The model under review builds one solid part; all positions refer to its coordinate system, in mm. Face numbers are marked on the shaded views. Round coordinates to 2 decimals unless told otherwise and drop trailing zeros. Order: outer loops, then holes, each group sorted by start corner. A loop starts at its lowest first (then second) coordinate and runs counter-clockwise, first axis right, second up. Notation, with made-up numbers: (-36.5, -36.75) -> (13.5, -36.75) arc R32 cw to (13.5, -2.75) -> close; hole circle Ø10 at (24.25, 47.5). An arc over 180 degrees is marked (long way). Return JSON: item names as keys, results as strings. Group by question number.
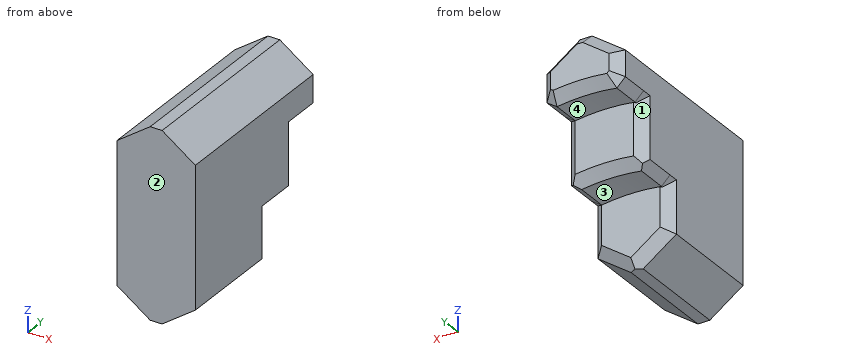
from build123d import *

# Parameters (mm, degrees)
EXTRUDE1_DEPTH     = 9.9822
CUT_EXTRUDE1_DEPTH = 36.749577377
SKETCH3_R          = 25.885731189
CUT_EXTRUDE2_DEPTH = 4.9022
SKETCH4_R          = 25.885731189
CUT_EXTRUDE3_DEPTH = 5.2578
CHAMFER1_SIZE      = 1.08172717
CHAMFER1_SIZE_2    = 1.27
CHAMFER2_SIZE      = 1.27
CHAMFER3_SIZE      = 1.27
CHAMFER4_SIZE      = 1.27


with BuildPart() as part:
    # Sketch1 → Extrude1 (new body)
    with BuildSketch(Plane(origin=(0, 0, 0), x_dir=(0, 0, -1), z_dir=(1, 0, 0))):
        Polygon((7.5692, 24.6888), (7.5692, 19.7866), (15.4432, 19.7866), (15.4432, 14.5288), (23.8506, 14.5288), (23.8506, 0), (0, 0), (0, 24.6888), align=None)
    extrude(amount=EXTRUDE1_DEPTH)

    # Sketch2 → Cut-Extrude1 (cut, through all)
    with BuildSketch(Plane(origin=(0, 24.6888, 0), x_dir=(1, 0, 0), z_dir=(0, 1, 0))):
        Polygon((0, 2.9972), (4.2291, 0), (0, 0), align=None)
        Polygon((9.9822, 2.9972), (9.9822, 0), (5.7531, 0), align=None)
        Polygon((0, 23.8506), (4.2291, 23.8506), (0, 20.8534), align=None)
        Polygon((9.9822, 20.8534), (9.9822, 23.8506), (5.7531, 23.8506), align=None)
    extrude(amount=-CUT_EXTRUDE1_DEPTH, mode=Mode.SUBTRACT)

    # Sketch3 → Cut-Extrude2 (cut)
    with BuildSketch(Plane(origin=(0, 24.6888, 0), x_dir=(1, 0, 0), z_dir=(0, 1, 0))):
        with Locations((4.9911, 32.9692)):
            Circle(SKETCH3_R)
    extrude(amount=-CUT_EXTRUDE2_DEPTH, mode=Mode.SUBTRACT)

    # Sketch4 → Cut-Extrude3 (cut)
    with BuildSketch(Plane(origin=(0, 19.7866, 0), x_dir=(1, 0, 0), z_dir=(0, 1, 0))):
        with Locations((4.9911, 40.8432)):
            Circle(SKETCH4_R)
    extrude(amount=-CUT_EXTRUDE3_DEPTH, mode=Mode.SUBTRACT)

    # Chamfer1
    # the kernel refuses this chamfer: 1.27, 1.08172717 mm, written as the material it takes off along each edge
    with BuildSketch(Plane(origin=(9.9822, 23.137823144, -15.4432), x_dir=(-0.9857782143008734, 0, 0.168051516535202), z_dir=(0, -1, 0))) as chamfer1_piece_1:
        with BuildLine():
            Line((1.303218251, 0), (CHAMFER1_SIZE * 0.168051516609, -CHAMFER1_SIZE * 0.985778214731))
            Line((CHAMFER1_SIZE * 0.168051516609, -CHAMFER1_SIZE * 0.985778214731), (0, 0))
            ThreePointArc((0, 0), (0.67003435, -0.008196065), (1.303218251, 0))
        make_face()
    extrude(amount=8.609023144, mode=Mode.SUBTRACT)
    with BuildSketch(Plane(origin=(9.9822, 28.040023144, -7.5692), x_dir=(0, 0, 1), z_dir=(0, -1, 0))) as chamfer1_piece_2:
        with BuildLine():
            Line((CHAMFER1_SIZE, 0), (0.219007803, 1.28468416))
            ThreePointArc((0.219007803, 1.28468416), (0.12067979, 0.659127904), (0, 0))
            Line((0, 0), (CHAMFER1_SIZE, 0))
        make_face()
    extrude(amount=8.253423144, mode=Mode.SUBTRACT)
    with BuildSketch(Plane(origin=(0, 27.954837395, -7.5692), x_dir=(0.9851028173062452, 0, 0.1719663901327771), z_dir=(0, -1, 0))) as chamfer1_piece_3:
        with BuildLine():
            Line((1.097600724, 0), (CHAMFER1_SIZE_2 * 0.171966390133, CHAMFER1_SIZE_2 * 0.985102817306))
            Line((CHAMFER1_SIZE_2 * 0.171966390133, CHAMFER1_SIZE_2 * 0.985102817306), (0, 0))
            ThreePointArc((0, 0), (0.563419729, 0.005814052), (1.097600724, 0))
        make_face()
    extrude(amount=8.168237395, mode=Mode.SUBTRACT)
    with BuildSketch(Plane(origin=(0, 23.052637395, -15.4432), x_dir=(0.985102817306246, 0, 0.17196639013277196), z_dir=(0, -1, 0))) as chamfer1_piece_4:
        with BuildLine():
            Line((1.097600724, 0), (CHAMFER1_SIZE_2 * 0.171966390133, CHAMFER1_SIZE_2 * 0.985102817306))
            Line((CHAMFER1_SIZE_2 * 0.171966390133, CHAMFER1_SIZE_2 * 0.985102817306), (0, 0))
            ThreePointArc((0, 0), (0.563419729, 0.005814052), (1.097600724, 0))
        make_face()
    extrude(amount=8.523837395, mode=Mode.SUBTRACT)

    # Chamfer2
    # the kernel refuses this chamfer: 1.27 mm, written as the material it takes off along each edge
    with BuildSketch(Plane(origin=(3.088405412, 24.6888, 1.88849226), x_dir=(0, -1, 0), z_dir=(0.8158799994392605, 0, -0.5782212608638604))) as chamfer2_piece_1:
        Polygon((CHAMFER2_SIZE, 0), (0, CHAMFER2_SIZE), (0, 0), align=None)
    extrude(amount=11.715557658, mode=Mode.SUBTRACT)
    with BuildSketch(Plane(origin=(0.963062605, 24.6888, 0), x_dir=(0, 0, -1), z_dir=(1, 0, 0))) as chamfer2_piece_2:
        Polygon((CHAMFER2_SIZE, 0), (0, -CHAMFER2_SIZE), (0, 0), align=None)
    extrude(amount=8.056074789, mode=Mode.SUBTRACT)
    with BuildSketch(Plane(origin=(-2.664694588, 24.6888, -4.88569226), x_dir=(0.5782212608638604, 0, -0.8158799994392603), z_dir=(0.8158799994392604, 0, 0.5782212608638605))) as chamfer2_piece_3:
        Polygon((CHAMFER2_SIZE, 0), (0, -CHAMFER2_SIZE), (0, 0), align=None)
    extrude(amount=11.715557658, mode=Mode.SUBTRACT)
    with BuildSketch(Plane(origin=(0, 24.6888, 0.268837395), x_dir=(1, 0, 0), z_dir=(0, 0, -1))) as chamfer2_piece_4:
        Polygon((CHAMFER2_SIZE, 0), (0, CHAMFER2_SIZE), (0, 0), align=None)
    extrude(amount=9.834074789, mode=Mode.SUBTRACT)
    with BuildSketch(Plane(origin=(3.390686755, 24.6888, -9.689886755), x_dir=(0.7071067811864264, 0, 0.7071067811866687), z_dir=(-0.7071067811866687, 0, 0.7071067811864264))) as chamfer2_piece_5:
        Polygon((CHAMFER2_SIZE, 0), (0, -CHAMFER2_SIZE), (0, 0), align=None)
    extrude(amount=8.061192589, mode=Mode.SUBTRACT)
    with BuildSketch(Plane(origin=(4.9911, 24.6888, -32.9692), x_dir=(-0.27423691753181434, 0, 0.9616621616049208), z_dir=(-0.9616621616049208, 0, -0.27423691753181434))) as chamfer2_piece_6:
        Polygon((25.885731189 + CHAMFER2_SIZE, 0), (25.885731189, -CHAMFER2_SIZE), (25.885731189, 0), align=None)
    revolve(axis=Axis((4.9911, 24.6888, -32.9692), (0, 1, 0)), revolution_arc=31.377850279, mode=Mode.SUBTRACT)
    with BuildSketch(Plane(origin=(12.693590923, 24.6888, -4.666659955), x_dir=(-0.5574990899678705, 0, 0.8301775500969635), z_dir=(-0.8301775500969636, 0, -0.5574990899678705))) as chamfer2_piece_7:
        Polygon((CHAMFER2_SIZE, 0), (0, -CHAMFER2_SIZE), (0, 0), align=None)
    extrude(amount=8.079556, mode=Mode.SUBTRACT)
    with BuildSketch(Plane(origin=(9.9822, 24.6888, 0.268837395), x_dir=(-1, 0, 0), z_dir=(0, 0, -1))) as chamfer2_piece_8:
        Polygon((CHAMFER2_SIZE, 0), (0, -CHAMFER2_SIZE), (0, 0), align=None)
    extrude(amount=10.022347619, mode=Mode.SUBTRACT)
    with BuildSketch(Plane(origin=(9.9822, 14.5288, -24.119437395), x_dir=(-1, 0, 0), z_dir=(0, 0, 1))) as chamfer2_piece_9_section:
        Polygon((CHAMFER2_SIZE, 0), (0, CHAMFER2_SIZE), (0, 0), align=None)
    chamfer2_piece_9 = extrude(amount=13.02400196, mode=Mode.PRIVATE)
    chamfer2_piece_9 = split(chamfer2_piece_9, bisect_by=Plane(origin=(5.465987334, 14.5288, -17.394299305), z_dir=(0.5574990901783627, 0, -0.8301775499556092)), keep=Keep.TOP, mode=Mode.PRIVATE)
    add(chamfer2_piece_9, mode=Mode.SUBTRACT)
    with BuildSketch(Plane(origin=(0, 14.5288, -10.907162605), x_dir=(1, 0, 0), z_dir=(0, 0, -1))) as chamfer2_piece_10_section:
        Polygon((CHAMFER2_SIZE, 0), (0, CHAMFER2_SIZE), (0, 0), align=None)
    chamfer2_piece_10 = extrude(amount=13.212274789, mode=Mode.PRIVATE)
    chamfer2_piece_10 = split(chamfer2_piece_10, bisect_by=Plane(origin=(-1.633018697, 14.5288, -12.540181303), z_dir=(-0.7071067811864264, 0, -0.7071067811866687)), keep=Keep.TOP, mode=Mode.PRIVATE)
    chamfer2_piece_10 = chamfer2_piece_10 - Plane(origin=(4.9911, 14.5288, -40.8432), x_dir=(1, 0, 0), z_dir=(0, 1, 0)) * Cylinder(25.885731189, 32, mode=Mode.PRIVATE)
    add(chamfer2_piece_10, mode=Mode.SUBTRACT)
    with BuildSketch(Plane(origin=(0, 14.5288, -10.907162605), x_dir=(1, 0, 0), z_dir=(0, 0, -1))) as chamfer2_piece_11_section:
        Polygon((CHAMFER2_SIZE, 0), (0, CHAMFER2_SIZE), (0, 0), align=None)
    chamfer2_piece_11 = extrude(amount=13.212274789, mode=Mode.PRIVATE)
    chamfer2_piece_11 = split(chamfer2_piece_11, bisect_by=Plane(origin=(-1.633018697, 14.5288, -12.540181303), z_dir=(0.7071067811864264, 0, 0.7071067811866687)), keep=Keep.TOP, mode=Mode.PRIVATE)
    chamfer2_piece_11 = chamfer2_piece_11 & Plane(origin=(4.9911, 14.5288, -40.8432), x_dir=(1, 0, 0), z_dir=(0, 1, 0)) * Cylinder(25.885731189, 32, mode=Mode.PRIVATE)
    add(chamfer2_piece_11, mode=Mode.SUBTRACT)
    with BuildSketch(Plane(origin=(0, 14.5288, -10.907162605), x_dir=(1, 0, 0), z_dir=(0, 0, -1))) as chamfer2_piece_12_section:
        Polygon((CHAMFER2_SIZE, 0), (0, CHAMFER2_SIZE), (0, 0), align=None)
    chamfer2_piece_12 = extrude(amount=13.212274789, mode=Mode.PRIVATE)
    chamfer2_piece_12 = split(chamfer2_piece_12, bisect_by=Plane(origin=(-1.633018697, 14.5288, -12.540181303), z_dir=(-0.7071067811864264, 0, -0.7071067811866687)), keep=Keep.TOP, mode=Mode.PRIVATE)
    chamfer2_piece_12 = chamfer2_piece_12 & Plane(origin=(4.9911, 14.5288, -40.8432), x_dir=(1, 0, 0), z_dir=(0, 1, 0)) * Cylinder(25.885731189, 32, mode=Mode.PRIVATE)
    add(chamfer2_piece_12, mode=Mode.SUBTRACT)
    with BuildSketch(Plane(origin=(0, 19.7866, -17.439237395), x_dir=(1, 0, 0), z_dir=(0, 0, 1))) as chamfer2_piece_13_section:
        Polygon((CHAMFER2_SIZE, 0), (0, -CHAMFER2_SIZE), (0, 0), align=None)
    chamfer2_piece_13 = extrude(amount=14.406074789, mode=Mode.PRIVATE)
    chamfer2_piece_13 = chamfer2_piece_13 & Plane(origin=(4.9911, 19.7866, -32.9692), x_dir=(1, 0, 0), z_dir=(0, 1, 0)) * Cylinder(25.885731189, 34, mode=Mode.PRIVATE)
    chamfer2_piece_13 = split(chamfer2_piece_13, bisect_by=Plane(origin=(5.570018697, 19.7866, -11.869218697), z_dir=(-0.7071067811864264, 0, -0.7071067811866687)), keep=Keep.TOP, mode=Mode.PRIVATE)
    add(chamfer2_piece_13, mode=Mode.SUBTRACT)
    with BuildSketch(Plane(origin=(0, 19.7866, -17.439237395), x_dir=(1, 0, 0), z_dir=(0, 0, 1))) as chamfer2_piece_14_section:
        Polygon((CHAMFER2_SIZE, 0), (0, -CHAMFER2_SIZE), (0, 0), align=None)
    chamfer2_piece_14 = extrude(amount=14.406074789, mode=Mode.PRIVATE)
    chamfer2_piece_14 = chamfer2_piece_14 - Plane(origin=(4.9911, 19.7866, -32.9692), x_dir=(1, 0, 0), z_dir=(0, 1, 0)) * Cylinder(25.885731189, 34, mode=Mode.PRIVATE)
    chamfer2_piece_14 = split(chamfer2_piece_14, bisect_by=Plane(origin=(5.570018697, 19.7866, -11.869218697), z_dir=(-0.7071067811864264, 0, -0.7071067811866687)), keep=Keep.TOP, mode=Mode.PRIVATE)
    add(chamfer2_piece_14, mode=Mode.SUBTRACT)
    with BuildSketch(Plane(origin=(0, 19.7866, -17.439237395), x_dir=(1, 0, 0), z_dir=(0, 0, 1))) as chamfer2_piece_15_section:
        Polygon((CHAMFER2_SIZE, 0), (0, -CHAMFER2_SIZE), (0, 0), align=None)
    chamfer2_piece_15 = extrude(amount=14.406074789, mode=Mode.PRIVATE)
    chamfer2_piece_15 = chamfer2_piece_15 & Plane(origin=(4.9911, 19.7866, -32.9692), x_dir=(1, 0, 0), z_dir=(0, 1, 0)) * Cylinder(25.885731189, 34, mode=Mode.PRIVATE)
    chamfer2_piece_15 = split(chamfer2_piece_15, bisect_by=Plane(origin=(5.570018697, 19.7866, -11.869218697), z_dir=(0.7071067811864264, 0, 0.7071067811866687)), keep=Keep.TOP, mode=Mode.PRIVATE)
    add(chamfer2_piece_15, mode=Mode.SUBTRACT)
    with BuildSketch(Plane(origin=(9.9822, 19.7866, -3.221435435), x_dir=(-1, 0, 0), z_dir=(0, 0, -1))) as chamfer2_piece_16_section:
        Polygon((CHAMFER2_SIZE, 0), (0, -CHAMFER2_SIZE), (0, 0), align=None)
    chamfer2_piece_16 = extrude(amount=14.406074789, mode=Mode.PRIVATE)
    chamfer2_piece_16 = split(chamfer2_piece_16, bisect_by=Plane(origin=(11.493797972, 19.7866, -5.472371309), z_dir=(0.5574990899678705, 0, -0.8301775500969636)), keep=Keep.TOP, mode=Mode.PRIVATE)
    add(chamfer2_piece_16, mode=Mode.SUBTRACT)

    # Chamfer3
    chamfer3_edges = [part.edges().sort_by_distance(p)[0] for p in [
        (7.23265, 14.5288, -22.80203003),
        (4.983681173, 19.7866, -14.957469874),
    ]]
    chamfer(chamfer3_edges, length=CHAMFER3_SIZE)

    # Chamfer4
    chamfer4_edges = [part.edges().sort_by_distance(p)[0] for p in [
        (2.581452238, 14.5288, -22.682897683),
    ]]
    chamfer(chamfer4_edges, length=CHAMFER4_SIZE)


solid = part.part
Item 1: Wall thickness on line 1 along Y through (x, z) = (6.5, -8); line 2 along Y through (x, z) = (3, -17.25); line 3 along Z through (x, y) = (3, 15.75): over which ranges is each line inside the solid? List them lowest first.
Item 2: Insertion check: pin 1 Ø2 at (x, z) = (6.5, -9.5) entering from +Y; pin 2 Ø2 at (x, z) = (3.5, -18) entering from +Y; pin 3 Ø1 at (y, z) = (12, -17.5) entering from -X; pin 4 Ø1.5 at (x, y) = (2.5, 7) entering from -Z. Each pin has a flat end and moves straight along its axis. Give the tip position at first contact, or say it passes through.
Item 3: The part is to be moulded in two halves that separate along X. For the marked faces 1, 2, 3 and 4, say which applies: +X half, -X half, draft (parallel to the pull), parting line (faces both ways), or undercut.
Item 4: Consider section B-B on z = -11. State the section outline as (x, y) points.
Item 5: Consider section C-C on y = 1.5. State the section outline as (x, z) points, plus the area to 3 significant figures.
Item 6: Consider section A-A on y = 20.75. State the section outline as (x, z) points.
Item 7: Consider section D-D on z = -18.25. State the section outline as (x, y) points, plus the area to 3 significant figures.
Values:
{
 "1": {"line 1": "0 to 19.79", "line 2": "0 to 14.53", "line 3": "-15.03 to -0.87"},
 "2": {"pin 1": "y = 19.79", "pin 2": "y = 14.53", "pin 3": "x = 0", "pin 4": "z = -23.16"},
 "3": {"face 1": "-X half", "face 2": "draft", "face 3": "undercut", "face 4": "undercut"},
 "4": {"outline": "(0, 0) -> (9.98, 0) -> (9.98, 18.52) -> (8.71, 19.79) -> (1.27, 19.79) -> (0, 18.52) -> close"},
 "5": {"outline": "(0, -20.85) -> (4.23, -23.85) -> (5.75, -23.85) -> (9.98, -20.85) -> (9.98, -3) -> (5.75, 0) -> (4.23, 0) -> (0, -3) -> close", "area": "213 mm^2"},
 "6": {"outline": "(0, -6.3) -> (1.08, -7.38) arc R25.89 cw to (8.7, -7.35) -> (9.98, -6.49) -> (9.98, -3) -> (5.75, 0) -> (4.23, 0) -> (0, -3) -> close"},
 "7": {"outline": "(0, 0) -> (9.98, 0) -> (9.98, 13.26) -> (8.71, 14.53) -> (1.27, 14.53) -> (0, 13.26) -> close", "area": "143 mm^2"}
}
